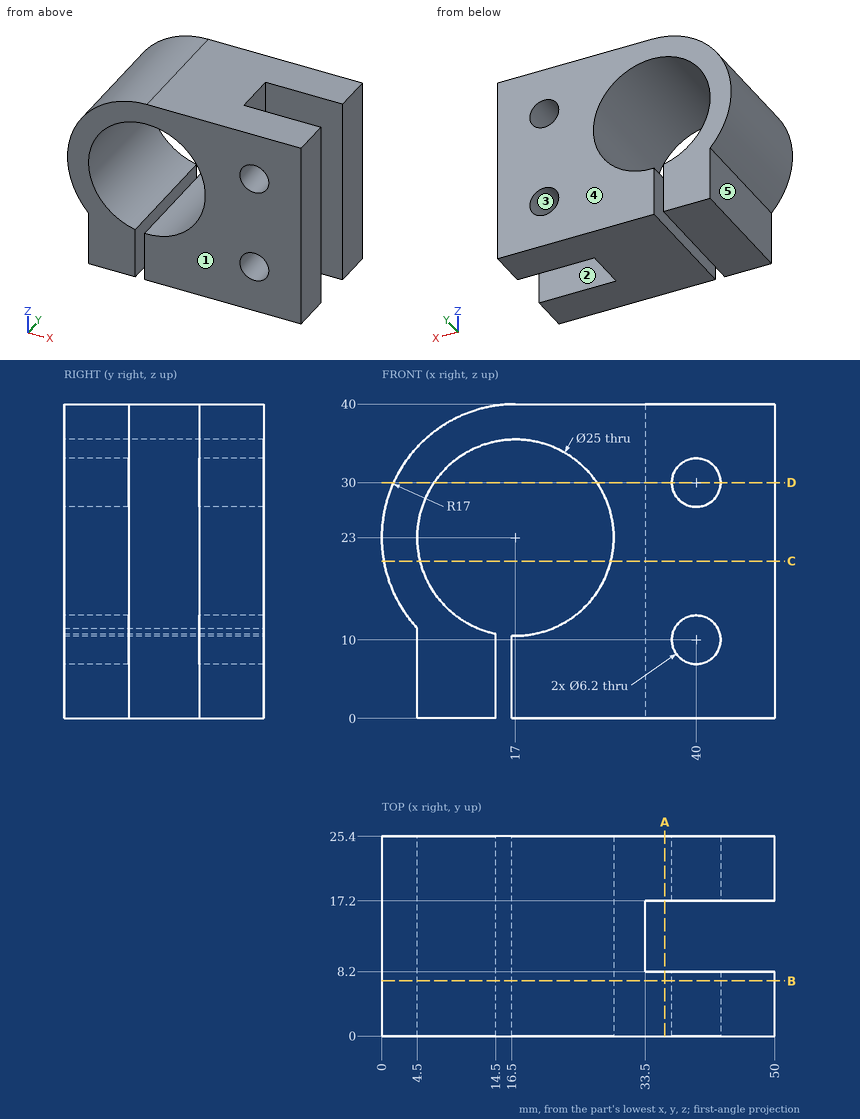
The drawing under review shows one solid part. Ordinate dimensions are in mm from its lowest x, y, z. A direction names the side the tool comes from. Round coordinates to 2 decimals unless told otherwise and drop trailing zeros. Loops run counter-clockwise (first coordinate to the right, second up) from the corner with the lowest first, then second, coordinate; pieces in that order, holes last. Notation, with made-up numbers: (-34.75, -36) - (13.25, -36) arc R20 cw to (13.25, -26) - close; hole circle Ø6 at (57, 23). An arc over 180 degrees is marked (long way). One line per item, written item: value. Start each with the question number.
1) Insertion check: pin 1 Ø5 at (x, y) = (11.5, 5.5) entering from +Z; pin 2 Ø10 at (x, z) = (40, 10) entering from -Y; pin 3 Ø5.5 at (y, z) = (7.5, 6.5) entering from -X; pin 4 Ø2 at (y, z) = (18, 17) entering from -X. Each pin has a flat end and moves straight along its axis. Give the tip position at first contact, or say it passes through.
2) To check wall thickness, follow L1, parallel to Z at x = 17, y = 10.75; L2, parallel to X at y = 20, z = 2; L3, parallel to X at y = 21, z = 30 (1 decimal). State the ranges of each line that lie inside material, in increasing order. Write a range as from..to.
3) Consider section B-B on y = 7. Give the boundary of the cut face in (x, z), then the cut area to 3 significant figures.
4) For the marked faces 1 and 2, list the 3-axis set-ups (+Z, -Z, +X, -X, +Y, -Y) from which the entire face can be reached by the end or side of a thin tool; tool diameter is ignored.
5) Consider section A-A on x = 36. Give the boundary of the cut face in (y, z), then the cut area to 3 significant figures.
6) Consider section D-D on z = 30. Give the boundary of the cut face in (x, y).
7) Consider section C-C on z = 20. Give the boundary of the cut face in (x, y) (1 decimal).
8) Draft analysis for pull direction X (two halves, no side actions). For the marked faces 3, 4 and 5, state which applies: +X half, -X half, draft (parallel to the pull), parting line (faces both ways), or undercut.
Reported:
1. pin 1: stops at z = 39.73
1. pin 2: stops at y = 0
1. pin 3: stops at x = 4.5
1. pin 4: stops at x = 0.75
2. L1: z = 0..10.5, 35.5..40
2. L2: x = 4.5..14.5, 16.5..50
2. L3: x = 1.5..6.6, 27.4..36.9, 43.1..50
3. outline: (4.5, 0) - (14.5, 0) - (14.5, 10.75) arc R12.5 cw (long way) to (16.5, 10.51) - (16.5, 0) - (50, 0) - (50, 40) - (17, 40) arc R17 ccw to (4.5, 11.48) - close; hole circle Ø6.2 at (40, 10); hole circle Ø6.2 at (40, 30)
3. area: 1,300 mm^2
4. face 1: +Z, -Z, +X, -X, -Y
4. face 2: +Z, -Z, +X
5. outline: (0, 0) - (8.2, 0) - (8.2, 40) - (0, 40) - close; (17.2, 0) - (25.4, 0) - (25.4, 40) - (17.2, 40) - close
5. area: 656 mm^2
6. outline: (1.51, 0) - (6.64, 0) - (6.64, 25.4) - (1.51, 25.4) - close; (27.36, 0) - (36.9, 0) - (36.9, 8.2) - (33.5, 8.2) - (33.5, 17.2) - (36.9, 17.2) - (36.9, 25.4) - (27.36, 25.4) - close; (43.1, 0) - (50, 0) - (50, 8.2) - (43.1, 8.2) - close; (43.1, 17.2) - (50, 17.2) - (50, 25.4) - (43.1, 25.4) - close
7. outline: (0.3, 0) - (4.9, 0) - (4.9, 25.4) - (0.3, 25.4) - close; (29.1, 0) - (50, 0) - (50, 8.2) - (33.5, 8.2) - (33.5, 17.2) - (50, 17.2) - (50, 25.4) - (29.1, 25.4) - close
8. face 3: undercut
8. face 4: draft
8. face 5: -X half
